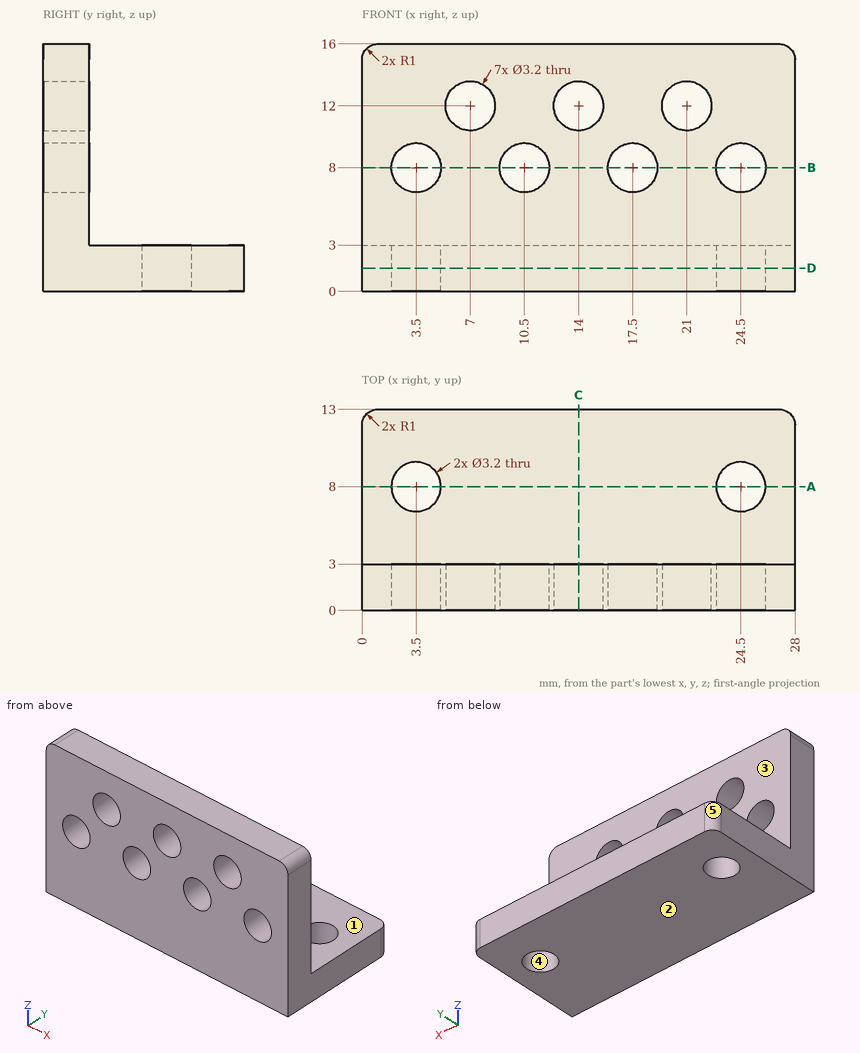
Source: three-view drawing plus pictorial views. Frame: mm from the lowest corner of the part. A direction names the side the tool comes from. Coordinates: 2 decimals unless noted, no trailing zeros. Loops run counter-clockwise (first coordinate to the right, second up) from the corner with the lowest first, then second, coordinate; pieces in that order, holes last. Notation, with made-up numbers: (-17, -29.75) - (40, -29.75) arc R15 ccw to (40, -10.75) - close; hole circle Ø9 at (87.5, 77). An arc over 180 degrees is marked (long way). One line per item, written item: value. Start each with the question number.
1. Set-up query: the marked faces 1 and 2. Return all of +Z, -Z, +X, -X, +Y, -Y with unobstructed straight access to the full face (end or side cutting, diameter ignored); none if empty.
2. Contact query for flat-ended pins moving along their axis: P1, Ø2.5, axis at x = 3.5, y = 8, coming from the +Z side; P2, Ø1.5, axis at x = 25, z = 14, coming from the +Y side. Output: stop coordinate, or through.
3. Section B-B (z = 8). Return the cut outline in (x, y).
4. Section A-A (y = 8). Return the cut outline in (x, z).
5. Ray query, L1, parallel to Z at x = 7, y = 1.5; L2, parallel to Y at x = 5, z = 8.75. Return the intervals inside material, ascending.
6. Section C-C (x = 14). Return the cut outline in (y, z), and give its area (3 significant figures).
7. Mould query, pull axis X, two halves, no side actions, for the marked faces 3, 4 and 5. Classes: pulls with the +X half, pulls with the -X half, needs draft (parallel to the pull), parting line crosses it, or undercut.
8. Section D-D (z = 1.5). Return the cut outline in (x, y), and give its area (3 significant figures).
Verdict:
1. face 1: +Z, +X, -X, +Y
1. face 2: -Z, +X, -X, +Y, -Y
2. P1: passes through
2. P2: stops at y = 3
3. outline: (0, 0) - (1.9, 0) - (1.9, 3) - (0, 3) - close; (5.1, 0) - (8.9, 0) - (8.9, 3) - (5.1, 3) - close; (12.1, 0) - (15.9, 0) - (15.9, 3) - (12.1, 3) - close; (19.1, 0) - (22.9, 0) - (22.9, 3) - (19.1, 3) - close; (26.1, 0) - (28, 0) - (28, 3) - (26.1, 3) - close
4. outline: (0, 0) - (1.9, 0) - (1.9, 3) - (0, 3) - close; (5.1, 0) - (22.9, 0) - (22.9, 3) - (5.1, 3) - close; (26.1, 0) - (28, 0) - (28, 3) - (26.1, 3) - close
5. L1: z = 0 to 10.4, 13.6 to 16
5. L2: y = 0 to 3
6. outline: (0, 0) - (13, 0) - (13, 3) - (3, 3) - (3, 10.4) - (0, 10.4) - close; (0, 13.6) - (3, 13.6) - (3, 16) - (0, 16) - close
6. area: 68.4 mm2
7. face 3: needs draft
7. face 4: undercut
7. face 5: pulls with the -X half
8. outline: (0, 0) - (28, 0) - (28, 12) arc R1 ccw to (27, 13) - (1, 13) arc R1 ccw to (0, 12) - close; hole circle Ø3.2 at (3.5, 8); hole circle Ø3.2 at (24.5, 8)
8. area: 347 mm2
